Verification items for this drawing (mm, ordinates from the low corner). A direction names the side the tool comes from. Give positions to 0.01 mm unless a question says otherwise; leave off trailing zeros. Loops run counter-clockwise (first coordinate to the right, second up) from the corner with the lowest first, then second, coordinate; pieces in that order, holes last. Notation, with made-up numbers: M 42.5,44.5 L 99.5,44.5 A8 cw 99.5,55.5 Z; hole C 70.5,-4 d11. An arc over 180 degrees is marked long. Answer in a Markdown table with one row per item.
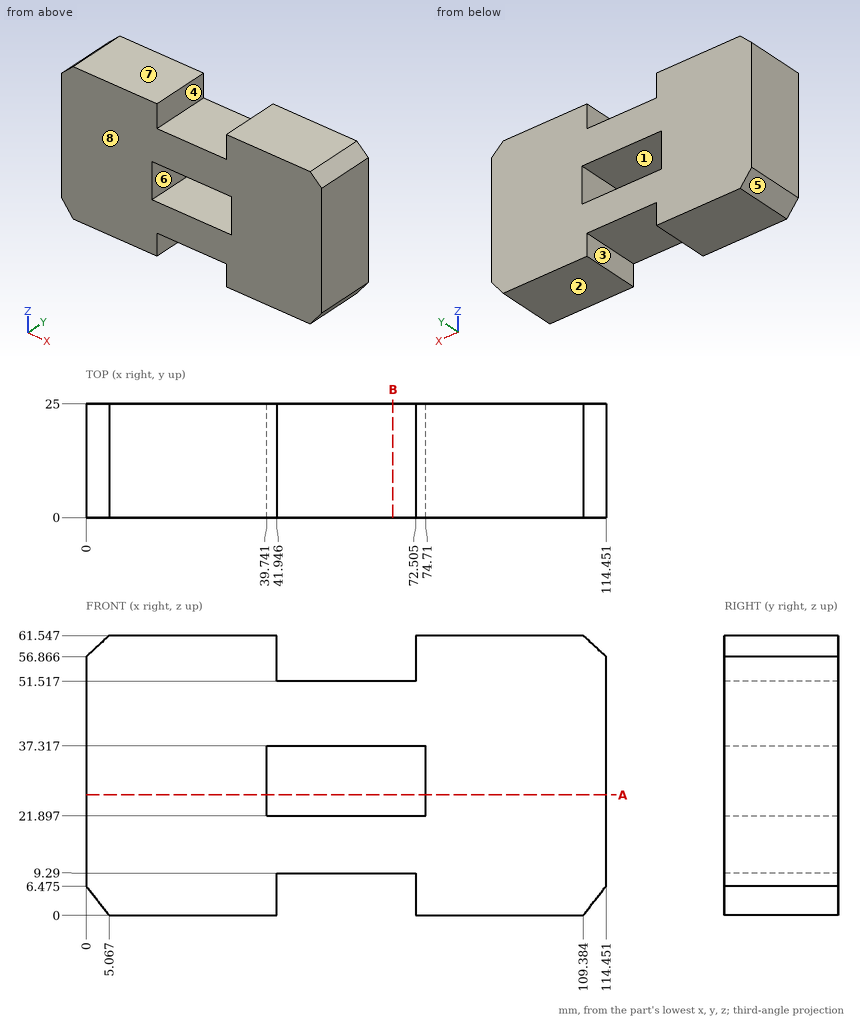
Item 1: Sectioned sample at B-B (x = 67.5). Record the cut outline in (y, z).
Reported:
| item | result |
|---|---|
| outline | M 0,9.29 L 25,9.29 L 25,21.9 L 0,21.9 Z; M 0,37.32 L 25,37.32 L 25,51.52 L 0,51.52 Z |
Item 2: Release check for a two-part mould opening along Z. For the marked faces 5, 6, 7 and 8 record: released by +Z, released by -Z, zero draft, split by the parting line, or undercut.
Reported:
| item | result |
|---|---|
| face 5 | released by -Z |
| face 6 | undercut |
| face 7 | released by +Z |
| face 8 | zero draft |
Item 3: Tool access check on the marked faces 1, 2, 3 and 4. Record the directions out of +Z, -Z, +X, -X, +Y, -Y that give a thin tool (end or side, any length) a straight path to the whole face; none if there is none.
Reported:
| item | result |
|---|---|
| face 1 | +Y, -Y |
| face 2 | -Z, +X, -X, +Y, -Y |
| face 3 | -Z, +Y, -Y |
| face 4 | +Z, +Y, -Y |
Item 4: Sectioned sample at A-A (z = 26.5). Record the cut outline in (x, y).
Reported:
| item | result |
|---|---|
| outline | M 0,0 L 39.74,0 L 39.74,25 L 0,25 Z; M 74.71,0 L 114.45,0 L 114.45,25 L 74.71,25 Z |
Item 5: Scan lines: L1, parallel to X at y = 4, z = 33; L2, parallel to Z at x = 57, y = 15.5; L3, parallel to X at y = 16.5, z = 58.5 (1 decimal). Record each from-to range of solid material in increasing order. Write a range as [from, to].
Reported:
| item | result |
|---|---|
| L1 | x = [0, 39.74], [74.71, 114.45] |
| L2 | z = [9.29, 21.9], [37.32, 51.52] |
| L3 | x = [1.8, 41.9], [72.5, 112.7] |
Item 6: Go/stop test with flat-tipped pins: pin 1 (3 mm diameter, centred on x = 48, z = 55, fed in from +Y); pin 2 (12.5 mm diameter, centred on x = 55.5, y = 11, fed in from -Z). Record where each tip stops, or that it passes through.
Reported:
| item | result |
|---|---|
| pin 1 | passes through |
| pin 2 | stops at z = 9.29 |
